```python
from build123d import *

# Parameters (mm, degrees)
EXTRUSION_BASE_SKETCH_W      = 230
EXTRUSION_BASE_SKETCH_H      = 20
EXTRUSION_BASE_SKETCH_R      = 2.65
EXTRUSION_BASE_EXTRUDE_DEPTH = 3


with BuildPart() as part:
    # Extrusion Base Sketch → Extrusion Base Extrude (new body)
    with BuildSketch(Plane.XY):
        with Locations((93.75, 7.5)):
            Rectangle(EXTRUSION_BASE_SKETCH_W, EXTRUSION_BASE_SKETCH_H)
        with Locations((-13.25, 7.5)):
            Circle(EXTRUSION_BASE_SKETCH_R, mode=Mode.SUBTRACT)
        with Locations((200.75, 7.5)):
            Circle(EXTRUSION_BASE_SKETCH_R, mode=Mode.SUBTRACT)
    extrude(amount=-EXTRUSION_BASE_EXTRUDE_DEPTH)


solid = part.part
```
Source: CAD feature listing. Evaluate the final solid. Frame: model axes, mm. Give positions to 0.01 mm unless a question says otherwise; leave off trailing zeros. Order: outer loops, then holes, each group sorted by start corner. A loop starts at its lowest first (then second) coordinate and runs counter-clockwise, first axis right, second up.
(1) Material intervals for line 1 along X through (y, z) = (6.25, -1); line 2 along Y through (x, z) = (200.75, -2); line 3 along X through (y, z) = (8.5, -0.7), sorted ascending.
(2) Pull-direction query (Y, two-part tool) for faces 1 (the face through (-10.8, 6.49, -1.48)), 2 (the face through (92, 8, 0)), 3 (the face through (203.2, 6.49, -1.48)); classes: +Y half, -Y half, draft (parallel to the pull), parting line (faces both ways), or undercut.
(3) Contact query for a flat-ended pin moving along its axis: P1, Ø5, axis at x = -13.25, y = 7.5, coming from the +Z side. Output: stop coordinate, or through.
(4) Section query A-A (y = 7.5). Return the cut outline in (x, z), plus the area to 3 significant figures.
(5) Section query B-B (x = 200.75). Return the cut outline in (y, z).
Outcome:
1. line 1: x = -21.25 to -15.59, -10.91 to 198.41, 203.09 to 208.75
1. line 2: y = -2.5 to 4.85, 10.15 to 17.5
1. line 3: x = -21.25 to -15.7, -10.8 to 198.3, 203.2 to 208.75
2. face 1: undercut
2. face 2: draft
2. face 3: undercut
3. P1: passes through
4. outline: (-21.25, -3) - (-15.9, -3) - (-15.9, 0) - (-21.25, 0) - close; (-10.6, -3) - (198.1, -3) - (198.1, 0) - (-10.6, 0) - close; (203.4, -3) - (208.75, -3) - (208.75, 0) - (203.4, 0) - close
4. area: 658 mm2
5. outline: (-2.5, -3) - (4.85, -3) - (4.85, 0) - (-2.5, 0) - close; (10.15, -3) - (17.5, -3) - (17.5, 0) - (10.15, 0) - close
